Can you work these out from the model? Positions are in its coordinate system, mm. A direction names the side the tool comes from. Give positions to 0.01 mm unless a question says otherwise; leave off trailing zeros. Order: outer loops, then holes, each group sorted by start corner. A loop starts at its lowest first (then second) coordinate and runs counter-clockwise, first axis right, second up. Notation, with made-up numbers: (-2.5, 7) -> (52.5, 7) arc R24 ccw to (52.5, 20) -> close; hole circle Ø1 at (-39, 3). An arc over 180 degrees is marked (long way). Answer as a JSON object with one key per item and string values.
```python
from build123d import *

# Parameters (mm, degrees)
SKETCH_1_R      = 3
SKETCH_1_R_2    = 1.2
EXTRUDE_1_DEPTH = 4.5
FILLET_1_R      = 8


with BuildPart() as part:
    # 草图1 → 凸台-拉伸1 (new body)
    with BuildSketch(Plane.XY):
        Polygon((-12.5, 0), (-18.5, 0), (-18.5, 42.034916596), (0, 60.534916596), (18.5, 42.034916596), (18.5, 0), (12.5, 0), (12.5, 35), (-12.5, 35), align=None)
        with Locations((0, 50.421397557)):
            Circle(SKETCH_1_R, mode=Mode.SUBTRACT)
        with Locations((-15.5, 5)):
            Circle(SKETCH_1_R_2, mode=Mode.SUBTRACT)
        with Locations((-15.5, 26)):
            Circle(SKETCH_1_R_2, mode=Mode.SUBTRACT)
        with Locations((15.5, 5)):
            Circle(SKETCH_1_R_2, mode=Mode.SUBTRACT)
        with Locations((15.5, 26)):
            Circle(SKETCH_1_R_2, mode=Mode.SUBTRACT)
    extrude(amount=EXTRUDE_1_DEPTH)

    # 圆角1
    fillet_1_edges = [part.edges().sort_by_distance(p)[0] for p in [
        (-18.5, 42.034916596, 2.25),
        (0, 60.534916596, 2.25),
        (18.5, 42.034916596, 2.25),
    ]]
    fillet(fillet_1_edges, radius=FILLET_1_R)


solid = part.part
```
1. For faces 1 (the face through (10.833, 49.702, 2.218)), 2 (the face through (12.5, 17, 2)), which set-ups out of +Z, -Z, +X, -X, +Y, -Y let a thin tool reach every point of the face, with its end or its side?
Worked answers:
{"face 1": "+Z, -Z, +X, +Y", "face 2": "+Z, -Z, -Y"}
2. If we section it at D-D on x = 15.5: Please give me the cut outline in (y, z).
Worked answers:
{"outline": "(0, 0) -> (3.8, 0) -> (3.8, 4.5) -> (0, 4.5) -> close; (6.2, 0) -> (24.8, 0) -> (24.8, 4.5) -> (6.2, 4.5) -> close; (27.2, 0) -> (45.03, 0) -> (45.03, 4.5) -> (27.2, 4.5) -> close"}
3. Will these pins go through, and if not, where does the flat tip stop? pin 1 Ø1.5 at (x, z) = (6.5, 0.5) entering from -Y; pin 2 Ø9.5 at (x, y) = (0, 50.42) entering from +Z.
Worked answers:
{"pin 1": "y = 35", "pin 2": "z = 4.5"}
4. If we section it at A-A on y = 26: Please give me the cut outline in (x, z), then the cut area to 3 significant figures.
Worked answers:
{"outline": "(-18.5, 0) -> (-16.7, 0) -> (-16.7, 4.5) -> (-18.5, 4.5) -> close; (-14.3, 0) -> (-12.5, 0) -> (-12.5, 4.5) -> (-14.3, 4.5) -> close; (12.5, 0) -> (14.3, 0) -> (14.3, 4.5) -> (12.5, 4.5) -> close; (16.7, 0) -> (18.5, 0) -> (18.5, 4.5) -> (16.7, 4.5) -> close", "area": "32.4 mm²"}
5. If we section it at C-C on z = 1.95: Please give me the cut outline in (x, y), then the cut area to 3 significant figures.
Worked answers:
{"outline": "(-18.5, 0) -> (-12.5, 0) -> (-12.5, 35) -> (12.5, 35) -> (12.5, 0) -> (18.5, 0) -> (18.5, 38.72) arc R8 ccw to (16.16, 44.38) -> (5.66, 54.88) arc R8 ccw to (-5.66, 54.88) -> (-16.16, 44.38) arc R8 ccw to (-18.5, 38.72) -> close; hole circle Ø2.4 at (-15.5, 5); hole circle Ø2.4 at (-15.5, 26); hole circle Ø6 at (0, 50.42); hole circle Ø2.4 at (15.5, 5); hole circle Ø2.4 at (15.5, 26)", "area": "960 mm²"}
6. If we section it at B-B on x = 0: Please give me the cut outline in (y, z).
Worked answers:
{"outline": "(35, 0) -> (47.42, 0) -> (47.42, 4.5) -> (35, 4.5) -> close; (53.42, 0) -> (57.22, 0) -> (57.22, 4.5) -> (53.42, 4.5) -> close"}
7. Please list where these lines run through material, in increasing order: L1, parallel to X at y = 14, z = 2.1; L2, parallel to Y at x = 0, z = 0.9; L3, parallel to X at y = 27, z = 2.05.
Worked answers:
{"L1": "-18.5 to -12.5, 12.5 to 18.5", "L2": "35 to 47.42, 53.42 to 57.22", "L3": "-18.5 to -16.16, -14.84 to -12.5, 12.5 to 14.84, 16.16 to 18.5"}
8. If we mould it in two halves opening along Y, with no side actions, what happens to faces 3 (the face through (-14.946, 24.935, 2.218)), 4 (the face through (-15, 0, 2)), 5 (the face through (-17.91, 41.74, 2.28))? For each: +Y half, -Y half, draft (parallel to the pull), parting line (faces both ways), or undercut.
Worked answers:
{"face 3": "undercut", "face 4": "-Y half", "face 5": "+Y half"}
